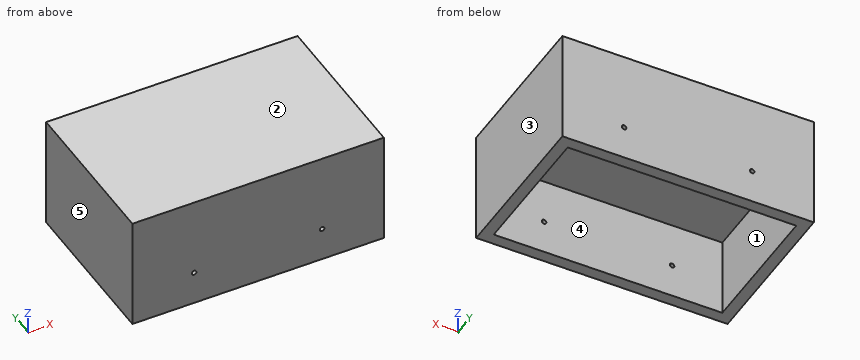
from build123d import *

# Parameters (mm, degrees)
SKETCH_1_W               = 110
SKETCH_1_H               = 70
EXTRUDE_1_DEPTH          = 50
SKETCH_3_W               = 100
SKETCH_3_H               = 60
CUT_EXTRUDE_1_DEPTH      = 35
SKETCH_4_R               = 1
CUT_EXTRUDE_2_DEPTH      = 40
CUT_EXTRUDE_2_DEPTH_BACK = 40


with BuildPart() as part:
    # 草圖1 → 填料-伸長1 (new body)
    with BuildSketch(Plane.XY):
        Rectangle(SKETCH_1_W, SKETCH_1_H)
    extrude(amount=EXTRUDE_1_DEPTH)

    # 草圖3 → 除料-伸長1 (cut)
    with BuildSketch(Plane.XY):
        Rectangle(SKETCH_3_W, SKETCH_3_H)
    extrude(amount=CUT_EXTRUDE_1_DEPTH, mode=Mode.SUBTRACT)

    # 草圖4 → 除料-伸長2 (cut, two sides)
    with BuildSketch(Plane(origin=(0, 0, 0), x_dir=(1, 0, 0), z_dir=(0, 1, 0))) as cut_extrude_2_sk:
        with Locations((28, -15)):
            Circle(SKETCH_4_R)
        with Locations((-28, -15)):
            Circle(SKETCH_4_R)
    extrude(amount=CUT_EXTRUDE_2_DEPTH, mode=Mode.SUBTRACT)
    extrude(cut_extrude_2_sk.sketch, amount=-CUT_EXTRUDE_2_DEPTH_BACK, mode=Mode.SUBTRACT)


solid = part.part
Verification items for the finished model (mm, model axes). Face numbers are marked on the shaded views. A direction names the side the tool comes from. Coordinates: 2 decimals unless noted, no trailing zeros. Write each loop counter-clockwise with the first axis right and the second up, starting at its lowest first coordinate (ties: lowest second). Pieces come first, ordered by that corner, then holes. Notation, with made-up numbers: M 64,-27.75 L 118,-27.75 A33 ccw 118,3.25 Z; hole C 77.25,4.5 d11. An arc over 180 degrees is marked long. Use CSV: the item, a comma, the result in double quotes.
Q1. Thickness scan on line 1 along X through (y, z) = (-32.2, 15); line 2 along Z through (x, y) = (-28, 31.3); line 3 along Y through (x, z) = (-30, 25). Record the ranges inside material, lowest first. Write a range as [from, to].
Computed values:
line 1,"[-55, -29], [-27, 27], [29, 55]"
line 2,"[0, 14], [16, 50]"
line 3,"[-35, -30], [30, 35]"
Q2. Section check C-C, the plane y = 9. Enter the section's corners in (x, z).
Computed values:
outline,"M -55,0 L -50,0 L -50,35 L 50,35 L 50,0 L 55,0 L 55,50 L -55,50 Z"
Q3. Mould release check, pull along X, two halves, no side actions. Record for the marked faces 1, 2 and 3: pulls with the +X half, pulls with the -X half, needs draft (parallel to the pull), parting line crosses it, or undercut.
Computed values:
face 1,"undercut"
face 2,"needs draft"
face 3,"pulls with the +X half"
Q4. Section check B-B, the plane x = -41. Enter the section's corners in (y, z), and give its area (3 significant figures).
Computed values:
outline,"M -35,0 L -30,0 L -30,35 L 30,35 L 30,0 L 35,0 L 35,50 L -35,50 Z"
area,"1,400 mm²"
Q5. Set-up check for the marked faces 4 and 5: record each of +Z, -Z, +X, -X, +Y, -Y from which the full face is reachable in a straight line by a thin tool's end or side.
Computed values:
face 4,"-Z"
face 5,"+Z, -Z, -X, +Y, -Y"
Q6. Go/stop test with a flat-tipped pin: P1, Ø18, axis at x = 9.5, y = -12, coming from the -Z side. Record where the tip stops, or that it passes through.
Computed values:
P1,"z = 35"
Q7. Section check A-A, the plane z = 6.5. Enter the section's corners in (x, y).
Computed values:
outline,"M -55,-35 L 55,-35 L 55,35 L -55,35 Z; hole M -50,-30 L 50,-30 L 50,30 L -50,30 Z"
